Verification items for the finished model (mm, model axes). A direction names the side the tool comes from. Coordinates: 2 decimals unless noted, no trailing zeros. Order: outer loops, then holes, each group sorted by start corner. A loop starts at its lowest first (then second) coordinate and runs counter-clockwise, first axis right, second up. Notation, with made-up numbers: M 56.25,74.25 L 69.25,74.25 A5 ccw 69.25,82.25 Z; hole C 41.5,-15.5 d3. An arc over 180 degrees is marked long. Return JSON: item names as keys, results as strings. Group by question number.
Q1. Go/stop test with a flat-tipped pin: pin 1 Ø2 at (x, y) = (-0.5, -3) entering from +Z. Record where the tip stops, or that it passes through.
Q2. Section check A-A, the plane z = 0. Enter the section's corners in (x, y), then the cut area to 3 significant figures.
Q3. Thickness scan on probe 1 along Z at (x, y) = (-0.3, 0); probe 2 along X at (y, z) = (-2.5, -6.5); probe 3 along X at (y, z) = (4, -4.75). Record the ranges inside material, lowest first.
Q4. Mould release check, pull along X, two halves, no side actions. Record for faces 3 (the face through (1.75, 0, -2)), 4 (the face through (-1, 3, 6)), 5 (the face through (0, -6, 0)), 6 (the face through (-1.504, -7.493, 0.33)): pulls with the +X half, pulls with the -X half, needs draft (parallel to the pull), parting line crosses it, or undercut.
Q5. Access from +Z, -Z, +X, -X, +Y, -Y to the whole of each face (thin tool, end or side, straight path). Record for faces 1 (the face through (1.496, -7.493, 0.33)), 2 (the face through (1, -3, 6)).
Q6. Section check D-D, the plane x = -0.05. Enter the section's corners in (y, z), then the cut area to 3 significant figures.
Q7. Section check C-C, the plane x = -1.45. Enter the section's corners in (y, z), then the cut area to 3 significant figures.
from build123d import *

# Parameters (mm, degrees)
FILLET1_R = 0.25


with BuildPart() as part:
    # Sketch1 → Revolve1 (revolve)
    with BuildSketch(Plane.XY):
        with BuildLine():
            Line((-1.75, 1), (1.75, 1))
            Line((1.75, 1), (1.75, 7.5))
            Line((1.75, 7.5), (1, 7.5))
            Line((1, 7.5), (1, 6.5))
            ThreePointArc((1, 6.5), (0.853553391, 6.146446609), (0.5, 6))
            Line((0.5, 6), (-0.5, 6))
            ThreePointArc((-0.5, 6), (-0.853553391, 6.146446609), (-1, 6.5))
            Line((-1, 6.5), (-1, 7.5))
            Line((-1, 7.5), (-1.75, 7.5))
            Line((-1.75, 7.5), (-1.75, 1))
        make_face()
    revolve(axis=Axis((0, 0, 0), (1, 0, 0)))

    # Fillet1
    fillet1_edges = [part.edges().sort_by_distance(p)[0] for p in [
        (1, -7.5, 0),
        (-1, -7.5, 0),
    ]]
    fillet(fillet1_edges, radius=FILLET1_R)


solid = part.part
Numbers:
{
 "1": {"pin 1": "stops at z = 7.14"},
 "2": {"outline": "M -1.75,-7.5 L -1.25,-7.5 A0.25 ccw -1,-7.25 L -1,-6.5 A0.5 cw -0.5,-6 L 0.5,-6 A0.5 cw 1,-6.5 L 1,-7.25 A0.25 ccw 1.25,-7.5 L 1.75,-7.5 L 1.75,-1 L -1.75,-1 Z; M -1.75,1 L 1.75,1 L 1.75,7.5 L 1.25,7.5 A0.25 ccw 1,7.25 L 1,6.5 A0.5 cw 0.5,6 L -0.5,6 A0.5 cw -1,6.5 L -1,7.25 A0.25 ccw -1.25,7.5 L -1.75,7.5 Z", "area": "39.7 mm2"},
 "3": {"probe 1": "z = -6 to -1, 1 to 6", "probe 2": "x = -1.75 to -1, 1 to 1.75", "probe 3": "x = -1.75 to -0.91, 0.91 to 1.75"},
 "4": {"face 3": "pulls with the +X half", "face 4": "undercut", "face 5": "undercut", "face 6": "needs draft"},
 "5": {"face 1": "+X, -X", "face 2": "none"},
 "6": {"outline": "C 0,0 d12; hole C 0,0 d2", "area": "110 mm2"},
 "7": {"outline": "C 0,0 d15; hole C 0,0 d2", "area": "174 mm2"}
}
